```python
from build123d import *

# Parameters (mm, degrees)
BOSS_EXTRUDE3_START = 4.25
BOSS_EXTRUDE3_DEPTH = 6
SKETCH3_R           = 1.575
CUT_EXTRUDE1_DEPTH  = 10


with BuildPart() as part:
    # Sketch2 → Boss-Extrude3 (new body)
    with BuildSketch(Plane.XY.offset(BOSS_EXTRUDE3_START)):
        with BuildLine():
            ThreePointArc((46.632238895, 16.118255038), (45.815068573, 16.097527081), (45, 16.035396523))
            ThreePointArc((45, 16.035396523), (38.72701102, 14.046548248), (33.771749201, 9.716272448))
            ThreePointArc((33.771749201, 9.716272448), (37.029755518, 5.335725192), (38.184673742, 0))
            Line((38.184673742, 0), (43.982238895, 0))
            ThreePointArc((43.982238895, 0), (44.758405925, 1.87383297), (46.632238895, 2.65))
            Line((46.632238895, 2.65), (46.632238895, 16.118255038))
        make_face()
        with BuildLine():
            ThreePointArc((33.771749201, -9.716272448), (38.72701102, -14.046548248), (45, -16.035396523))
            ThreePointArc((45, -16.035396523), (45.815068573, -16.097527081), (46.632238895, -16.118255038))
            Line((46.632238895, -16.118255038), (46.632238895, -2.65))
            ThreePointArc((46.632238895, -2.65), (44.758405925, -1.87383297), (43.982238895, 0))
            Line((43.982238895, 0), (38.184673742, 0))
            ThreePointArc((38.184673742, 0), (37.029755518, -5.335725192), (33.771749201, -9.716272448))
        make_face()
        with BuildLine():
            ThreePointArc((38.184673742, 0), (37.029755518, 5.335725192), (33.771749201, 9.716272448))
            ThreePointArc((33.771749201, 9.716272448), (31.350112109, 5.123938556), (30.513983858, 0))
            Line((30.513983858, 0), (38.184673742, 0))
        make_face()
        with BuildLine():
            ThreePointArc((30.513983858, 0), (31.350112109, -5.123938556), (33.771749201, -9.716272448))
            ThreePointArc((33.771749201, -9.716272448), (37.029755518, -5.335725192), (38.184673742, 0))
            Line((38.184673742, 0), (30.513983858, 0))
        make_face()
        with BuildLine():
            ThreePointArc((56.268821721, 12.920310248), (51.708915452, 15.297892031), (46.632238895, 16.118255038))
            Line((46.632238895, 16.118255038), (46.632238895, 2.65))
            ThreePointArc((46.632238895, 2.65), (48.506071865, 1.87383297), (49.282238895, 0))
            Line((49.282238895, 0), (50.616596945, 0))
            ThreePointArc((50.616596945, 0), (52.091474062, 7.051277576), (56.268821721, 12.920310248))
        make_face()
        with BuildLine():
            Line((46.632238895, -2.65), (46.632238895, -16.118255038))
            ThreePointArc((46.632238895, -16.118255038), (51.708915452, -15.297892031), (56.268821721, -12.920310248))
            ThreePointArc((56.268821721, -12.920310248), (52.091474062, -7.051277576), (50.616596945, 0))
            Line((50.616596945, 0), (49.282238895, 0))
            ThreePointArc((49.282238895, 0), (48.506071865, -1.87383297), (46.632238895, -2.65))
        make_face()
        with BuildLine():
            add(Edge.make_bspline(
                [(67.5, 17.578928476), (65.61016752, 17.502615465), (60.634413429, 17.271238409), (53.13057404, 16.789010877), (47.524682176, 16.292383273), (45, 16.035396523)],
                knots=[0.381536428, 0.381536428, 0.381536428, 0.381536428, 0.390812303, 0.405965006, 0.418410632, 0.418410632, 0.418410632, 0.418410632], degree=3))
            ThreePointArc((45, 16.035396523), (45.815068573, 16.097527081), (46.632238895, 16.118255038))
            ThreePointArc((46.632238895, 16.118255038), (51.708915452, 15.297892031), (56.268821721, 12.920310248))
            ThreePointArc((56.268821721, 12.920310248), (61.469163108, 16.250714817), (67.5, 17.578928476))
        make_face()
        with BuildLine():
            ThreePointArc((46.632238895, -16.118255038), (45.815068573, -16.097527081), (45, -16.035396523))
            add(Edge.make_bspline(
                [(45, -16.035396523), (47.524682176, -16.292383273), (53.13057404, -16.789010877), (60.634413429, -17.271238409), (65.61016752, -17.502615465), (67.5, -17.578928476)],
                knots=[0.581589368, 0.581589368, 0.581589368, 0.581589368, 0.594034994, 0.609187697, 0.618463572, 0.618463572, 0.618463572, 0.618463572], degree=3))
            ThreePointArc((67.5, -17.578928476), (61.469163108, -16.250714817), (56.268821721, -12.920310248))
            ThreePointArc((56.268821721, -12.920310248), (51.708915452, -15.297892031), (46.632238895, -16.118255038))
        make_face()
    extrude(amount=BOSS_EXTRUDE3_DEPTH)

    # Sketch3 → Cut-Extrude1 (cut)
    with BuildSketch(Plane.XY.offset(10.25)):
        with Locations((43.902744235, -5.9)):
            Circle(SKETCH3_R)
        with Locations((43.982238895, 5.9)):
            Circle(SKETCH3_R)
    extrude(amount=-CUT_EXTRUDE1_DEPTH, mode=Mode.SUBTRACT)


solid = part.part
```
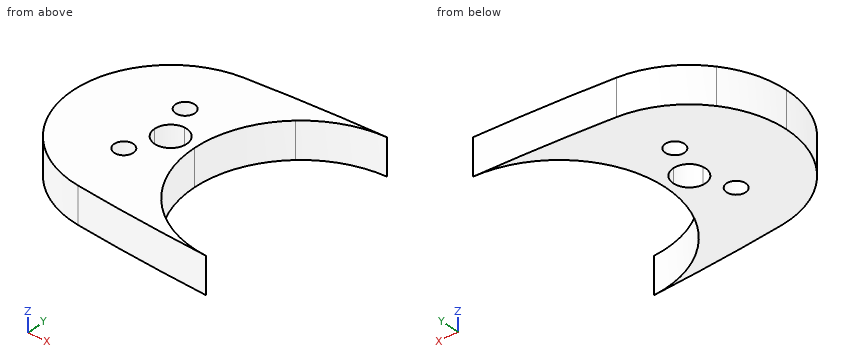
Here's how the part is built. I have some questions about the finished solid (model axes, mm). Round coordinates to 2 decimals unless told otherwise and drop trailing zeros. Order: outer loops, then holes, each group sorted by start corner. A loop starts at its lowest first (then second) coordinate and runs counter-clockwise, first axis right, second up. Notation, with made-up numbers: (0.5, 54.25) -> (36.5, 54.25) arc R28 cw to (36.5, 74.25) -> close; hole circle Ø8 at (-15.75, 53.5). An arc over 180 degrees is marked (long way). Use a Markdown table: item, result. Add a question column.
(1) Suppose I cut it at B-B, the plane z = 9.25. Count the separate pieces of the cut face and the enclosed holes in it, and give its area (3 significant figures).
(2) I need wall thicknesses on line 1 along Y through (x, z) = (43, 5); line 2 along Y through (x, z) = (65, 7.75); line 3 along X through (y, z) = (1.5, 5.5). Which ranges of each line are inside material? Lowest first, please.
(3) Suppose I cut it at C-C, the plane y = -5.9. Please give me the cut outline in (x, z), and give its area (3 significant figures).
(4) For pin 1 Ø3 at (y, z) = (13, 6.5) entering from -X; pin 2 Ø2 at (x, z) = (50.5, 9) entering from -Y; pin 3 Ø1 at (y, z) = (-4, 6.5) entering from -X; pin 4 Ø1.9 at (x, y) = (43.98, 5.9) entering from +Z, each with a flat end and sliding along its axis, tell me the tip position at first contact or that it passes through.
(5) Suppose I cut it at A-A, the plane y = -1.5. Please give me the cut outline in (x, z), and give its area (3 significant figures).
(6) Suppose I cut it at D-D, the plane y = -10.5. Please give me the cut outline in (x, z), and give its area (3 significant figures).
Verdict:
| question | item | result |
|---|---|---|
| 1 | separate pieces | 1 |
| 1 | enclosed holes | 3 |
| 1 | area | 618 mm2 |
| 2 | line 1 | -15.7 to -7.19, -4.61 to 4.67, 7.13 to 15.7 |
| 2 | line 2 | -17.47 to -17.3, 17.3 to 17.47 |
| 2 | line 3 | 30.58 to 44.45, 48.82 to 50.68 |
| 3 | outline | (31.63, 4.25) -> (42.33, 4.25) -> (42.33, 10.25) -> (31.63, 10.25) -> close; (45.48, 4.25) -> (51.64, 4.25) -> (51.64, 10.25) -> (45.48, 10.25) -> close |
| 3 | area | 101 mm2 |
| 4 | pin 1 | x = 35.34 |
| 4 | pin 2 | y = -16.63 |
| 4 | pin 3 | x = 30.9 |
| 4 | pin 4 | through |
| 5 | outline | (30.58, 4.25) -> (44.45, 4.25) -> (44.45, 10.25) -> (30.58, 10.25) -> close; (48.82, 4.25) -> (50.68, 4.25) -> (50.68, 10.25) -> (48.82, 10.25) -> close |
| 5 | area | 94.4 mm2 |
| 6 | outline | (34.4, 4.25) -> (54.09, 4.25) -> (54.09, 10.25) -> (34.4, 10.25) -> close |
| 6 | area | 118 mm2 |
